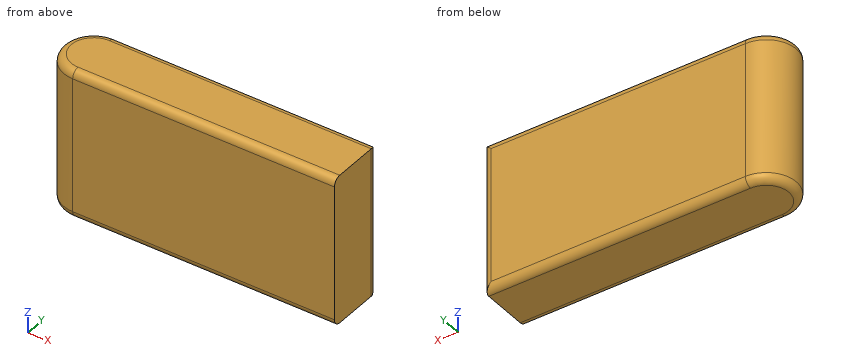
from build123d import *

# Parameters (mm, degrees)
EXTRUDE_1_DEPTH = 20
FILLET_1_R      = 1


with BuildPart() as part:
    # Эскиз1 → Бобышка-Вытянуть1 (new body)
    with BuildSketch(Plane.XY):
        with BuildLine():
            Line((17.5, -4), (-17.5, -4))
            ThreePointArc((-17.5, -4), (-21.5, 0), (-17.5, 4))
            Line((-17.5, 4), (17.5, 4))
            Line((17.5, 4), (17.5, -4))
        make_face()
    extrude(amount=EXTRUDE_1_DEPTH)

    # Скругление1
    fillet_1_edges = [part.edges().sort_by_distance(p)[0] for p in [
        (0, 4, 20),
        (-21.5, 0, 20),
        (0, 4, 0),
        (0, -4, 0),
        (-21.5, 0, 0),
        (17.5, 4, 10),
        (0, -4, 20),
    ]]
    fillet(fillet_1_edges, radius=FILLET_1_R)


solid = part.part
Could you check a few things on this model? Use its own coordinates, in mm. Give positions to 0.01 mm unless a question says otherwise; leave off trailing zeros. Order: outer loops, then holes, each group sorted by start corner. A loop starts at its lowest first (then second) coordinate and runs counter-clockwise, first axis right, second up. Notation, with made-up numbers: (54.5, 81) -> (84.5, 81) arc R19 ccw to (84.5, 89) -> close; hole circle Ø3 at (-6.5, 88). An arc over 180 degrees is marked (long way). Answer in a Markdown table with one row per item. Add a question column.
Item 1: I'm going to push a flat-ended pin straight in: P1, Ø1.5, axis at y = 1.5, z = 17, coming from the -X side. Where does the tip first touch, or does it pass through?
Item 2: Please list where these lines run through material, in increasing order: probe 1 along X at (y, z) = (1, 5.75); probe 2 along X at (y, z) = (1.25, 18.25); probe 3 along Z at (x, y) = (-2, -3.5).
Item 3: Imagine slicing it at A-A (z = 14.25). List the corners of the cut face in (x, y) for me, and give its area (3 significant figures).
Result:
| question | item | result |
|---|---|---|
| 1 | P1 | x = -21.43 |
| 2 | probe 1 | -21.37 to 17.5 |
| 2 | probe 2 | -21.3 to 17.5 |
| 2 | probe 3 | 0.13 to 19.87 |
| 3 | outline | (-17.5, -4) -> (17.5, -4) -> (17.5, 3) arc R1 ccw to (16.5, 4) -> (-17.5, 4) arc R4 ccw to start |
| 3 | area | 305 mm2 |
